Check sheet for the drawn part. Datum: minimum x, y, z corner. Units: mm. Coordinates: 2 decimals unless noted, no trailing zeros. Order: outer loops, then holes, each group sorted by start corner. A loop starts at its lowest first (then second) coordinate and runs counter-clockwise, first axis right, second up. Notation, with made-up numbers: M 2,19.25 L 23,19.25 A29 ccw 23,43.25 Z; hole C 6.5,13 d11. An arc over 180 degrees is marked long. Return JSON: item names as keys, results as strings. Group by question number.
Q1. Section check C-C, the plane z = 1.15. Enter the section's corners in (x, y), then the cut area to 3 significant figures.
Q2. Go/stop test with a flat-tipped pin: pin 1 Ø8 at (x, y) = (79, 30) entering from -Z. Record where the tip stops, or that it passes through.
Q3. Section check A-A, the plane y = 33. Enter the section's corners in (x, z), then the cut area to 3 significant figures.
Q4. Section check D-D, the plane y = 6. Enter the section's corners in (x, z), then the cut area to 3 significant figures.
Q5. Section check B-B, the plane x = 16.5. Enter the section's corners in (y, z).
Q6. Thickness scan on probe 1 along Y at (x, z) = (45, 2.2); probe 2 along X at (y, z) = (29, 3.3); probe 3 along Y at (x, z) = (107, 2.3). Record the ranges inside material, lowest first.
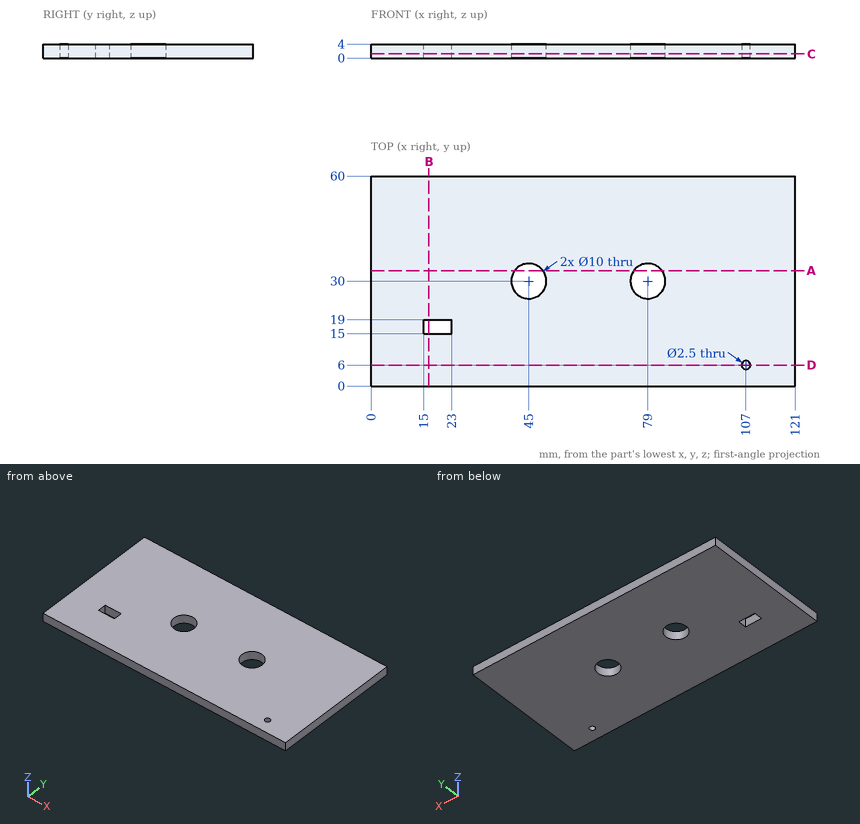
Numbers:
{
 "1": {"outline": "M 0,0 L 121,0 L 121,60 L 0,60 Z; hole M 15,15 L 23,15 L 23,19 L 15,19 Z; hole C 45,30 d10; hole C 79,30 d10; hole C 107,6 d2.5", "area": "7,070 mm2"},
 "2": {"pin 1": "passes through"},
 "3": {"outline": "M 0,0 L 41,0 L 41,4 L 0,4 Z; M 49,0 L 75,0 L 75,4 L 49,4 Z; M 83,0 L 121,0 L 121,4 L 83,4 Z", "area": "420 mm2"},
 "4": {"outline": "M 0,0 L 105.75,0 L 105.75,4 L 0,4 Z; M 108.25,0 L 121,0 L 121,4 L 108.25,4 Z", "area": "474 mm2"},
 "5": {"outline": "M 0,0 L 15,0 L 15,4 L 0,4 Z; M 19,0 L 60,0 L 60,4 L 19,4 Z"},
 "6": {"probe 1": "y = 0 to 25, 35 to 60", "probe 2": "x = 0 to 40.1, 49.9 to 74.1, 83.9 to 121", "probe 3": "y = 0 to 4.75, 7.25 to 60"}
}
